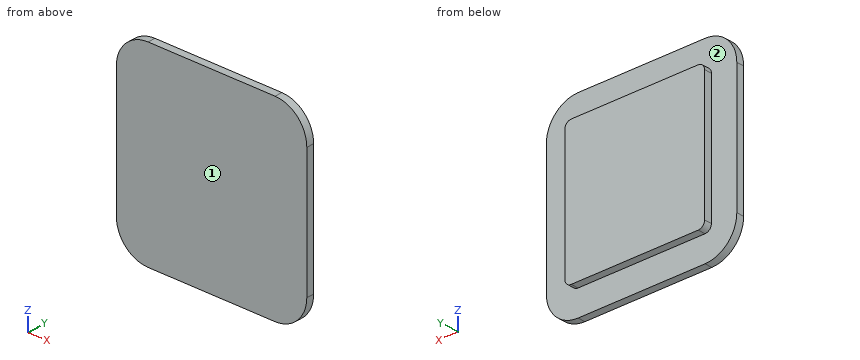
from build123d import *

# Parameters (mm, degrees)
SKETCH_1_W      = 15
SKETCH_1_H      = 15
EXTRUDE_1_DEPTH = 0.6
FILLET_1_R      = 2.5
SKETCH_2_W      = 11
SKETCH_2_H      = 11
EXTRUDE_2_DEPTH = 0.6
FILLET_2_R      = 0.5


with BuildPart() as part:
    # 草图1 → 凸台-拉伸1 (new body)
    with BuildSketch(Plane(origin=(0, 0, 0), x_dir=(1, 0, 0), z_dir=(0, 1, 0))):
        with Locations((53.495024876, 28.718905473)):
            Rectangle(SKETCH_1_W, SKETCH_1_H)
    extrude(amount=EXTRUDE_1_DEPTH)

    # 圆角1
    fillet_1_edges = [part.edges().sort_by_distance(p)[0] for p in [
        (45.995024876, 0.3, -36.218905473),
        (60.995024876, 0.3, -36.218905473),
        (60.995024876, 0.3, -21.218905473),
        (45.995024876, 0.3, -21.218905473),
    ]]
    fillet(fillet_1_edges, radius=FILLET_1_R)

    # 草图2 → 凸台-拉伸2 (add)
    with BuildSketch(Plane(origin=(0, 0.6, 0), x_dir=(1, 0, 0), z_dir=(0, 1, 0))):
        with Locations((53.495024876, 28.718905473)):
            Rectangle(SKETCH_2_W, SKETCH_2_H)
    extrude(amount=EXTRUDE_2_DEPTH)

    # 圆角2
    fillet_2_edges = [part.edges().sort_by_distance(p)[0] for p in [
        (47.995024876, 0.9, -34.218905473),
        (47.995024876, 0.9, -23.218905473),
        (58.995024876, 0.9, -23.218905473),
        (58.995024876, 0.9, -34.218905473),
    ]]
    fillet(fillet_2_edges, radius=FILLET_2_R)


solid = part.part
Can you work these out from the model? Positions are in its coordinate system, mm. Face numbers are marked on the shaded views. A direction names the side the tool comes from. Coordinates: 2 decimals unless noted, no trailing zeros. Loops run counter-clockwise (first coordinate to the right, second up) from the corner with the lowest first, then second, coordinate; pieces in that order, holes last. Notation, with made-up numbers: (53.5, -19.5) - (89.5, -19.5) arc R18 cw to (89.5, -0.5) - close; hole circle Ø7 at (55, 3.5). An arc over 180 degrees is marked (long way). Answer as a JSON object with one key per item and string values. Group by question number.
Item 1: For pin 1 (0.7 mm diameter, centred on x = 55, y = 1, fed in from +Z), with a flat end and sliding along its axis, tell me the tip position at first contact or that it passes through.
Item 2: If we section it at C-C (x = 47): List the corners of the cut face in (y, z) for me.
Item 3: If we section it at B-B (z = -31): List the corners of the cut face in (x, y) for me, plus the area to 3 significant figures.
Item 4: If we section it at D-D (z = -22.25): List the corners of the cut face in (x, y) for me, plus the area to 3 significant figures.
Item 5: If we section it at A-A (y = 0.3): List the corners of the cut face in (x, z) for me.
Item 6: If I drill on L1, parallel to Y at x = 48.75, z = -22.75; L2, parallel to X at y = 1.05, z = -30.75; L3, parallel to Z at x = 57, y = 0.95, over which ranges is the centre line in solid material (lowest first)? Write a range as from..to.
Item 7: On a 3-axis mill with a long thin cutter (end or side, diameter ignored), from which of +Z, -Z, +X, -X, +Y, -Y can I reach the whole of each face in a straight line? I mean the marked faces 1 and 2. Say none if no direction works.
Returned:
{
 "1": {"pin 1": "stops at z = -23.22"},
 "2": {"outline": "(0, -35.72) - (0.6, -35.72) - (0.6, -21.72) - (0, -21.72) - close"},
 "3": {"outline": "(46, 0) - (61, 0) - (61, 0.6) - (59, 0.6) - (59, 1.2) - (48, 1.2) - (48, 0.6) - (46, 0.6) - close", "area": "15.6 mm²"},
 "4": {"outline": "(46.47, 0) - (60.52, 0) - (60.52, 0.6) - (46.47, 0.6) - close", "area": "8.43 mm²"},
 "5": {"outline": "(46, -33.72) arc R2.5 ccw to (48.5, -36.22) - (58.5, -36.22) arc R2.5 ccw to (61, -33.72) - (61, -23.72) arc R2.5 ccw to (58.5, -21.22) - (48.5, -21.22) arc R2.5 ccw to (46, -23.72) - close"},
 "6": {"L1": "y = 0..0.6", "L2": "x = 48..59", "L3": "z = -34.22..-23.22"},
 "7": {"face 1": "+Z, -Z, +X, -X, -Y", "face 2": "+Y"}
}
